Design review of the part built by this model. Coordinates are the model's own, in mm. A direction names the side the tool comes from. Coordinates: 2 decimals unless noted, no trailing zeros. Write each loop counter-clockwise with the first axis right and the second up, starting at its lowest first coordinate (ties: lowest second). Pieces come first, ordered by that corner, then holes. Notation, with made-up numbers: M 33.25,31 L 53.25,31 A18 ccw 53.25,60 Z; hole C 68,4.25 d9. An arc over 180 degrees is marked long. One line per question, with ' | ' between items.
from build123d import *

# Parameters (mm, degrees)
F1_DEPTH = 10
F2_R     = 0.1
F3_SIZE  = 2
F4_R     = 2


with BuildPart() as f1:
    # F0 (on Top) → F1 (new body)
    with BuildSketch(Plane.XY):
        Polygon((6.5, 20), (6.5, 70), (0, 70), (-6.5, 70), (-6.5, 20), (-11, 20), (-11, 11), (0, 0), (11, 11), (11, 20), align=None)
    extrude(amount=F1_DEPTH)

    # F2
    f2_edges = [f1.edges().sort_by_distance(p)[0] for p in [
        (0, 0, 5),
    ]]
    fillet(f2_edges, radius=F2_R)

    # F3
    f3_edges = [f1.edges().sort_by_distance(p)[0] for p in [
        (-11, 20, 5),
        (11, 20, 5),
    ]]
    chamfer(f3_edges, length=F3_SIZE)

    # F4
    f4_edges = [f1.edges().sort_by_distance(p)[0] for p in [
        (9, 20, 5),
        (11, 18, 5),
        (-9, 20, 5),
        (-11, 18, 5),
    ]]
    fillet(f4_edges, radius=F4_R)


solid = f1.part
1. Insertion check: pin 1 Ø1.5 at (x, z) = (-5, 8.5) entering from -Y; pin 2 Ø0.8 at (x, z) = (-7.5, 6) entering from +Y; pin 3 Ø3 at (y, z) = (39, 5.5) entering from +X; pin 4 Ø3 at (x, z) = (-1, 6) entering from -Y. Each pin has a flat end and moves straight along its axis. Give the tip position at first contact, or say it passes through.
Answer sheet:
pin 1: y = 4.25 | pin 2: y = 20 | pin 3: x = 6.5 | pin 4: y = 0.04
2. To check wall thickness, follow line 1 along X through (y, z) = (48, 9.5); line 2 along Y through (x, z) = (-1, 5.5); line 3 along Y through (x, z) = (-5.75, 6.75). State the ranges of each line that lie inside material, in increasing order. Write a range as [from, to].
Answer sheet:
line 1: [-6.5, 6.5] | line 2: [1, 70] | line 3: [5.75, 70]
3. Take a section at B-B (x = 5.75). Write out the cut boundary in (y, z).
Answer sheet:
outline: M 5.75,0 L 70,0 L 70,10 L 5.75,10 Z
4. Take a section at C-C (y = 5.5). Write out the cut boundary in (x, z).
Answer sheet:
outline: M -5.5,0 L 5.5,0 L 5.5,10 L -5.5,10 Z
5. Tool access review of faces 1 (the face through (0, 36, 10)), 2 (the face through (-7, 20, 5)), 3 (the face through (6.5, 45, 5)): name each direction out of +Z, -Z, +X, -X, +Y, -Y from which nothing blocks a thin tool from reaching the whole face with its end or side.
Answer sheet:
face 1: +Z, +X, -X, +Y, -Y | face 2: +Z, -Z, -X, +Y | face 3: +Z, -Z, +X, +Y
6. Take a section at A-A (z = 5.25). Write out the cut boundary in (x, y), then the cut area to 3 significant figures.
Answer sheet:
outline: M -11,11 L -0.07,0.07 A0.1 ccw 0.07,0.07 L 11,11 L 11,17.17 A2 ccw 10.41,18.59 L 9.59,19.41 A2 ccw 8.17,20 L 6.5,20 L 6.5,70 L -6.5,70 L -6.5,20 L -8.17,20 A2 ccw -9.59,19.41 L -10.41,18.59 A2 ccw -11,17.17 Z | area: 965 mm^2
